from build123d import *

# Parameters (mm, degrees)
CROQUIS1_W                 = 55
CROQUIS1_H                 = 25
SALIENTE_EXTRUIR1_DEPTH    = 2.5
CROQUIS7_W                 = 51
CROQUIS7_H                 = 21
CROQUIS7_W_2               = 47
CROQUIS7_H_2               = 17
SALIENTE_EXTRUIR4_DEPTH    = 3
REDONDEO2_R                = 3
CROQUIS8_W                 = 12
CROQUIS8_H                 = 17
CORTAR_EXTRUIR5_DEPTH      = 11
CORTAR_EXTRUIR5_DEPTH_BACK = 8
CROQUIS9_W                 = 6
CROQUIS9_H                 = 5
CORTAR_EXTRUIR6_DEPTH      = 8
CROQUIS11_R                = 2.5
CORTAR_EXTRUIR8_DEPTH      = 3.5
CROQUIS12_W                = 51
CROQUIS12_H                = 21
CROQUIS12_W_2              = 50.4
CROQUIS12_H_2              = 20.4
CORTAR_EXTRUIR11_DEPTH     = 3


with BuildPart() as part:
    # Croquis1 → Saliente-Extruir1 (new body)
    with BuildSketch(Plane.XY):
        Rectangle(CROQUIS1_W, CROQUIS1_H)
    extrude(amount=SALIENTE_EXTRUIR1_DEPTH)

    # Croquis7 → Saliente-Extruir4 (add)
    with BuildSketch(Plane.XY.offset(2.5)):
        Rectangle(CROQUIS7_W, CROQUIS7_H)
        Rectangle(CROQUIS7_W_2, CROQUIS7_H_2, mode=Mode.SUBTRACT)
    extrude(amount=SALIENTE_EXTRUIR4_DEPTH)

    # Redondeo2
    redondeo2_edges = [part.edges().sort_by_distance(p)[0] for p in [
        (-27.5, -12.5, 1.25),
        (-27.5, 12.5, 1.25),
        (27.5, 12.5, 1.25),
        (27.5, -12.5, 1.25),
    ]]
    fillet(redondeo2_edges, radius=REDONDEO2_R)

    # Croquis8 → Cortar-Extruir5 (cut, two sides)
    with BuildSketch(Plane.XY.offset(2.5)) as cortar_extruir5_sk:
        with Locations((-20.225004992, 0)):
            Rectangle(CROQUIS8_W, CROQUIS8_H)
    extrude(amount=CORTAR_EXTRUIR5_DEPTH, mode=Mode.SUBTRACT)
    extrude(cortar_extruir5_sk.sketch, amount=-CORTAR_EXTRUIR5_DEPTH_BACK, mode=Mode.SUBTRACT)

    # Croquis9 → Cortar-Extruir6 (cut)
    with BuildSketch(Plane(origin=(0, 0, 0), x_dir=(-1, 0, 0), z_dir=(0, 0, -1))):
        with Locations((-24.5, 0)):
            Rectangle(CROQUIS9_W, CROQUIS9_H)
    extrude(amount=-CORTAR_EXTRUIR6_DEPTH, mode=Mode.SUBTRACT)

    # Croquis11 → Cortar-Extruir8 (cut, through all)
    with BuildSketch(Plane.XY.offset(2.5)):
        with Locations((-3.5, 6)):
            Circle(CROQUIS11_R)
        with Locations((17.5, -6)):
            Circle(CROQUIS11_R)
    extrude(amount=-CORTAR_EXTRUIR8_DEPTH, mode=Mode.SUBTRACT)

    # Croquis12 → Cortar-Extruir11 (cut)
    with BuildSketch(Plane.XY.offset(5.5)):
        Rectangle(CROQUIS12_W, CROQUIS12_H)
        Rectangle(CROQUIS12_W_2, CROQUIS12_H_2, mode=Mode.SUBTRACT)
    extrude(amount=-CORTAR_EXTRUIR11_DEPTH, mode=Mode.SUBTRACT)


solid = part.part
Source: CAD feature listing. Evaluate the final solid. Frame: model axes, mm. A direction names the side the tool comes from. Give positions to 0.01 mm unless a question says otherwise; leave off trailing zeros. Write each loop counter-clockwise with the first axis right and the second up, starting at its lowest first coordinate (ties: lowest second). Pieces come first, ordered by that corner, then holes. Notation, with made-up numbers: (36, 82.5) -> (84, 82.5) arc R10 ccw to (84, 88.5) -> close; hole circle Ø1 at (16, -26.75). An arc over 180 degrees is marked (long way). Return JSON: item names as keys, results as strings. Group by question number.
1. Material intervals for line 1 (X direction, y = -6, z = 0.9) (3 decimals); line 2 (X direction, y = 6, z = 1.1) (3 decimals); line 3 (Y direction, x = 17.5, z = 1.45), sorted ascending. Write a range as from..to.
2. Section C-C, the plane y = 4. Output: boundary loops of the cut face in (x, z) (3 decimals), then the cut area to 3 significant figures.
3. Section A-A, the plane x = -18. Output: boundary loops of the cut face in (y, z).
4. Section D-D, the plane z = 4.5. Output: boundary loops of the cut face in (x, y), then the cut area to 3 significant figures.
5. Section B-B, the plane y = 0.5. Output: boundary loops of the cut face in (x, z) (3 decimals).
6. Access query for faces 5 (the face through (21.5, 0, 1)), 6 (the face through (4, 0, 2.5)), 7 (the face through (-7, -8.5, 3)), 8 (the face through (-14.225, 0, 1)). Directions: +Z, -Z, +X, -X, +Y, -Y. A direction counts if a zero-diameter tool reaches every point of the face in a straight line with its end or side. Return the directions, or none.
7. Mould query, pull axis Y, two halves, no side actions, for faces 1 (the face through (0, -10.2, 4)), 2 (the face through (26.6, 11.64, 1.27)), 3 (the face through (23.5, -6, 4)), 4 (the face through (-2, 11, 2.5)). Classes: +Y half, -Y half, draft (parallel to the pull), parting line (faces both ways), or undercut.
8. Pin query (flat end, axial travel): pin 1 Ø4 at (x, y) = (5, -5.5) entering from +Z; pin 2 Ø3 at (x, y) = (17.5, -6) entering from -Z; pin 3 Ø2.5 at (x, z) = (0.5, 4.5) entering from -Y; pin 4 Ø0.9 at (y, z) = (-5.5, 4.5) entering from -X. Return the tip coordinate at first contact, or that it passes through.
Determined:
{
 "1": {"line 1": "x = -27.5..-26.225, -14.225..15, 20..27.5", "line 2": "x = -27.5..-26.225, -14.225..-6, -1..27.5", "line 3": "y = -12.5..-8.5, -3.5..12.5"},
 "2": {"outline": "(-27.5, 0) -> (-26.225, 0) -> (-26.225, 2.5) -> (-27.5, 2.5) -> close; (-14.225, 0) -> (-5, 0) -> (-5, 2.5) -> (-14.225, 2.5) -> close; (-2, 0) -> (27.5, 0) -> (27.5, 2.5) -> (25.2, 2.5) -> (25.2, 5.5) -> (23.5, 5.5) -> (23.5, 2.5) -> (-2, 2.5) -> close", "area": "105 mm2"},
 "3": {"outline": "(-12.5, 0) -> (-8.5, 0) -> (-8.5, 5.5) -> (-10.2, 5.5) -> (-10.2, 2.5) -> (-12.5, 2.5) -> close; (8.5, 0) -> (12.5, 0) -> (12.5, 2.5) -> (10.2, 2.5) -> (10.2, 5.5) -> (8.5, 5.5) -> close"},
 "4": {"outline": "(-25.2, -10.2) -> (25.2, -10.2) -> (25.2, -2.5) -> (23.5, -2.5) -> (23.5, -8.5) -> (-25.2, -8.5) -> close; (-25.2, 8.5) -> (23.5, 8.5) -> (23.5, 2.5) -> (25.2, 2.5) -> (25.2, 10.2) -> (-25.2, 10.2) -> close", "area": "192 mm2"},
 "5": {"outline": "(-27.5, 0) -> (-26.225, 0) -> (-26.225, 2.5) -> (-27.5, 2.5) -> close; (-14.225, 0) -> (21.5, 0) -> (21.5, 2.5) -> (-14.225, 2.5) -> close"},
 "6": {"face 5": "+Z, -Z, +X", "face 6": "+Z, -X", "face 7": "+Z", "face 8": "+Z, -Z"},
 "7": {"face 1": "-Y half", "face 2": "+Y half", "face 3": "undercut", "face 4": "draft"},
 "8": {"pin 1": "stops at z = 2.5", "pin 2": "passes through", "pin 3": "stops at y = -10.2", "pin 4": "stops at x = 23.5"}
}
